The model under review builds one solid part; all positions refer to its coordinate system, in mm. Face numbers are marked on the shaded views. A direction names the side the tool comes from. Round coordinates to 2 decimals unless told otherwise and drop trailing zeros. Order: outer loops, then holes, each group sorted by start corner. A loop starts at its lowest first (then second) coordinate and runs counter-clockwise, first axis right, second up. Notation, with made-up numbers: (50, 15.5) - (82, 15.5) arc R14 cw to (82, 30.5) - close; hole circle Ø10 at (-10, -1.5). An arc over 180 degrees is marked (long way). One line per question, with ' | ' between items. Start each with the question number.
Item 1: Add section C-C on x = 16. State the section outline as (y, z) points, and give its area (3 significant figures).
Item 2: For L1, parallel to X at y = -1.75, z = 0; L2, parallel to X at y = -7.5, z = 6; L3, parallel to Z at x = 0, y = 10, list the stretches that pass through material, from the lowest coordinate up. Write a range as [from, to].
Item 3: Add section D-D on z = -16. State the section outline as (x, y) points.
Item 4: Draft analysis for pull direction Y (two halves, no side actions). For the marked faces 3, 4 and 5, state which applies: +Y half, -Y half, draft (parallel to the pull), parting line (faces both ways), or undercut.
Item 5: Tool access review of the marked faces 1 and 2: name each direction out of +Z, -Z, +X, -X, +Y, -Y from which nothing blocks a thin tool from reaching the whole face with its end or side.
Item 6: Insertion check: pin 1 Ø3.5 at (x, z) = (0, 16) entering from +Y; pin 2 Ø6 at (x, z) = (11.5, 13.5) entering from +Y; pin 3 Ø1 at (y, z) = (13.5, 6) entering from -X; pin 4 Ø5 at (y, z) = (18, 6.5) entering from -X. Each pin has a flat end and moves straight along its axis. Give the tip position at first contact, or say it passes through.
Item 7: Add section A-A on z = 0. State the section outline as (x, y) points.
Item 8: Add section B-B on y = -5.5. State the section outline as (x, z) points.
from build123d import *

# Parameters (mm, degrees)
SKETCH1_R           = 10.5
BOSS_EXTRUDE1_DEPTH = 25
SKETCH4_R           = 20
BOSS_EXTRUDE2_DEPTH = 10
SKETCH5_R           = 6.75
CUT_EXTRUDE1_DEPTH  = 46
SKETCH6_W           = 2.8
SKETCH6_H           = 2.9
BOSS_EXTRUDE3_DEPTH = 35
SKETCH7_R           = 2
CUT_EXTRUDE2_DEPTH  = 10
SKETCH8_R           = 2
CUT_EXTRUDE3_DEPTH  = 20


with BuildPart() as part:
    # Sketch1 → Boss-Extrude1 (new body)
    with BuildSketch(Plane(origin=(0, 0, 0), x_dir=(1, 0, 0), z_dir=(0, 1, 0))):
        with Locations(Location((0, 0, 0), (0, 0, 270))):
            Circle(SKETCH1_R)
    extrude(amount=BOSS_EXTRUDE1_DEPTH)

    # Sketch4 → Boss-Extrude2 (add)
    with BuildSketch(Plane.XZ):
        with Locations(Location((0, 0, 0), (0, 0, 270))):
            Circle(SKETCH4_R)
    extrude(amount=BOSS_EXTRUDE2_DEPTH)

    # Sketch5 → Cut-Extrude1 (cut, through all)
    with BuildSketch(Plane(origin=(0, 25, 0), x_dir=(1, 0, 0), z_dir=(0, 1, 0))):
        with Locations(Location((0, 0, 0), (0, 0, 270))):
            Circle(SKETCH5_R)
    extrude(amount=-CUT_EXTRUDE1_DEPTH, mode=Mode.SUBTRACT)

    # Sketch6 → Boss-Extrude3 (add, through all)
    with BuildSketch(Plane(origin=(0, 25, 0), x_dir=(1, 0, 0), z_dir=(0, 1, 0))):
        with Locations((0, -6.75)):
            Rectangle(SKETCH6_W, SKETCH6_H)
    extrude(amount=-BOSS_EXTRUDE3_DEPTH)

    # Sketch7 → Cut-Extrude2 (cut)
    with BuildSketch(Plane.XZ.offset(10)):
        with Locations(Location((0, 16, 0), (0, 0, 270))):
            Circle(SKETCH7_R)
        with Locations(Location((16, 0, 0), (0, 0, 270))):
            Circle(SKETCH7_R)
        with Locations(Location((0, -16, 0), (0, 0, 270))):
            Circle(SKETCH7_R)
        with Locations(Location((-16, 0, 0), (0, 0, 270))):
            Circle(SKETCH7_R)
    extrude(amount=-CUT_EXTRUDE2_DEPTH, mode=Mode.SUBTRACT)

    # Sketch8 → Cut-Extrude3 (cut)
    with BuildSketch(Plane.XY):
        with Locations((0, 17.687279486)):
            Circle(SKETCH8_R)
    extrude(amount=-CUT_EXTRUDE3_DEPTH, mode=Mode.SUBTRACT)


solid = part.part
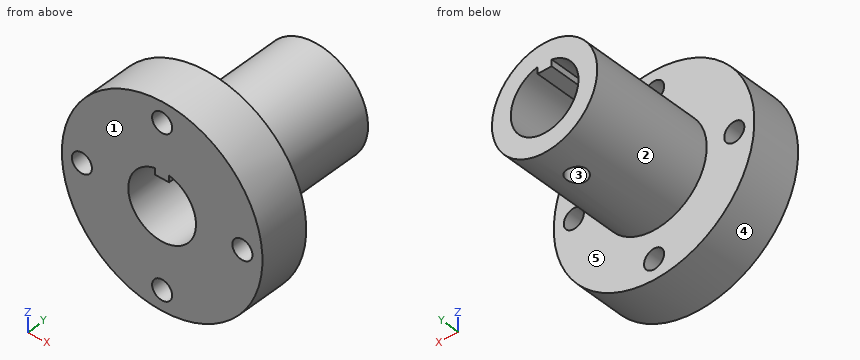
Determined:
1) outline: (-10, -12) - (0, -12) - (0, -2) - (-10, -2) - close; (-10, 2) - (0, 2) - (0, 12) - (-10, 12) - close | area: 200 mm2
2) L1: [-20, -18], [-14, -6.75], [6.75, 14], [18, 20] | L2: [-19.08, -3.09], [-1.4, 1.4], [3.09, 19.08] | L3: [-10.5, -6.75], [5.3, 10.5]
3) outline: (-12, -10) - (-2, -10) - (-2, 0) - (-12, 0) - close; (2, -10) - (12, -10) - (12, 0) - (2, 0) - close
4) face 3: undercut | face 4: draft | face 5: +Y half
5) face 1: +Z, -Z, +X, -X, -Y | face 2: +Y
6) pin 1: through | pin 2: y = 0 | pin 3: x = -8.94 | pin 4: x = -9.71
7) outline: (-20, -10) - (-18, -10) - (-18, 0) - (-20, 0) - close; (-14, -10) - (-6.75, -10) - (-6.75, 25) - (-10.5, 25) - (-10.5, 0) - (-14, 0) - close; (6.75, -10) - (14, -10) - (14, 0) - (10.5, 0) - (10.5, 25) - (6.75, 25) - close; (18, -10) - (20, -10) - (20, 0) - (18, 0) - close
8) outline: circle Ø40 at (0, 0); hole circle Ø4 at (-16, 0); hole circle Ø4 at (0, -16); hole circle Ø4 at (0, 16); hole (-1.4, 5.3) - (-1.4, 6.6) arc R6.75 ccw (long way) to (1.4, 6.6) - (1.4, 5.3) - close; hole circle Ø4 at (16, 0)
